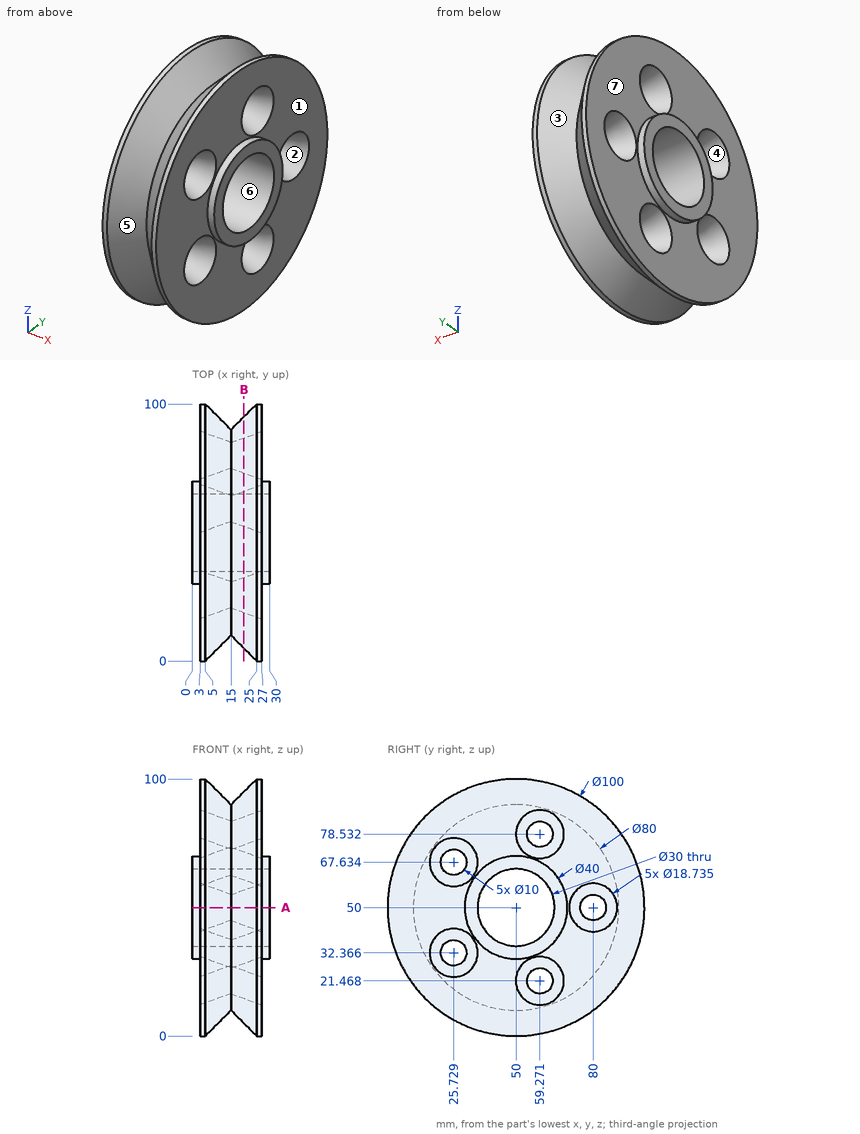
Geometry: see drawing. Coordinates: mm, zero at the bounding-box minimum. A direction names the side the tool comes from. Round coordinates to 2 decimals unless told otherwise and drop trailing zeros. Write each loop counter-clockwise with the first axis right and the second up, starting at its lowest first coordinate (ties: lowest second). Pieces come first, ordered by that corner, then holes. Notation, with made-up numbers: M 6.5,-31.75 L 43.5,-31.75 A26 ccw 43.5,7.25 Z; hole C 63.25,-6.5 d1. An arc over 180 degrees is marked long. Answer as a JSON object with one key per item and string values. Group by question number.
(1) First-contact query: pin 1 (12 mm diameter, centred on x = 13.5, z = 23, fed in from +Y) (1 decimal); pin 2 (3 mm diameter, centred on x = 25.5, y = 40, fed in from +Z); pin 3 (4 mm diameter, centred on x = 14, y = 78, fed in from -Z) (1 decimal). Flat tips, straight axial feed; report the tip coordinate or a pass-through.
(2) Mould query, pull axis Y, two halves, no side actions, for the marked faces 1, 2, 3 and 4. Classes: +Y half, -Y half, draft (parallel to the pull), parting line (faces both ways), or undercut.
(3) Section query A-A on z = 50. Output: boundary loops of the cut face in (x, y), then the cut area to 4 significant figures.
(4) Section query B-B on x = 20. State how many separate pieces and enclosed holes the cut face has, then the cut area to 3 significant figures.
(5) Ray query, line 1 (Z direction, x = 6.75, y = 25) (1 decimal); line 2 (Y direction, x = 7.25, z = 50); line 3 (Y direction, x = 23, z = 50). Return the intervals inside material, ascending. Write a range as [from, to].
(6) Reachability of the marked faces 5, 6 and 7 from +Z, -Z, +X, -X, +Y, -Y: full face, straight path, thin tool, end or side. Return the list, or none.
Computed values:
{
 "1": {"pin 1": "y = 90.1", "pin 2": "z = 99.27", "pin 3": "z = 16.9"},
 "2": {"face 1": "draft", "face 2": "undercut", "face 3": "parting line", "face 4": "undercut"},
 "3": {"outline": "M 0,30 L 3,30 L 3,0 L 5,0 L 15,10 L 25,0 L 27,0 L 27,30 L 30,30 L 30,35 L 0,35 Z; M 0,65 L 30,65 L 30,70 L 27,70 L 27,70.63 L 15,75 L 3,70.63 L 3,70 L 0,70 Z; M 3,89.37 L 15,85 L 27,89.37 L 27,100 L 25,100 L 15,90 L 5,100 L 3,100 Z", "area": "1,195 mm^2"},
 "4": {"separate pieces": "1", "enclosed holes": "6", "area": "4,920 mm^2"},
 "5": {"line 1": "[8.7, 24.4], [40.3, 59.7], [75.6, 91.3]", "line 2": "[2.25, 35], [65, 72.18], [87.82, 97.75]", "line 3": "[2, 35], [65, 72.09], [87.91, 98]"},
 "6": {"face 5": "none", "face 6": "+X, -X", "face 7": "-X"}
}
